Geometry check sheet. Reference: the model listing, model coordinates, mm. A direction names the side the tool comes from. Round coordinates to 2 decimals unless told otherwise and drop trailing zeros. Order: outer loops, then holes, each group sorted by start corner. A loop starts at its lowest first (then second) coordinate and runs counter-clockwise, first axis right, second up. Notation, with made-up numbers: (5.5, 47.5) - (56.5, 47.5) arc R21 ccw to (56.5, 83.5) - close; hole circle Ø2 at (9.25, 89.25). An arc over 180 degrees is marked (long way). Use a Markdown table: item, result. Add a question column.
(1) Section check A-A on z = 10.5. Record the boundary of the cut face in (x, y).
(2) Section check B-B on z = 8. Record the boundary of the cut face in (x, y).
(3) Thickness scan on line 1 along Z through (x, y) = (-7, -20); line 2 along Z through (x, y) = (-6.5, -34.25); line 3 along X through (y, z) = (-23, 2.5). Record the ranges inside material, lowest first. Write a range as [from, to].
(4) Mould release check, pull along Y, two halves, no side actions. Record for faces 3 (the face through (-6.44, -37.03, 6.76)), 4 (the face through (-5.53, -17.68, 4.18)), 5 (the face through (0, -22, 5)): released by +Y, released by -Y, zero draft, split by the parting line, or undercut.
(5) Access from +Z, -Z, +X, -X, +Y, -Y to the whole of each face (thin tool, end or side, straight path). Record for faces 1 (the face through (-5.39, -20.03, 1.01)), 2 (the face through (-8, -21.98, 5.31)).
(6) Gauge pin test, flat ends, axial feed: P1, Ø2, axis at x = -8, z = 4.5, coming from the -Y side; P2, Ø1.5, axis at x = -10, z = 6.5, coming from the -Y side; P3, Ø3, axis at x = -10, y = -34, coming from the +Z side. Record the tip position at first contact, or that the pin passes through.
```python
from build123d import *

# Parameters (mm, degrees)
F0_R     = 5.8053181287
F2_ANGLE = 20
F4_ANGLE = 10
F5_R     = 1.4002438662


with BuildPart() as f2:
    # F0 (on Right) → F2 (revolve)
    with BuildSketch(Plane.YZ):
        with BuildLine():
            Line((-32.5852286816, 0), (-12.5, 0))
            Line((-12.5, 0), (-11.0429839557, 5.8568340727))
            Line((-11.0429839557, 5.8568340727), (-30.835461438, 13.2508232685))
            ThreePointArc((-30.835461438, 13.2508232685), (-35.4357693129, 12.6748361661), (-37.5852286816, 8.5669878109))
            Line((-37.5852286816, 8.5669878109), (-37.5852286816, 5))
            ThreePointArc((-37.5852286816, 5), (-36.1207625875, 1.4644660941), (-32.5852286816, 0))
        make_face()
        with Locations((-31.1660505831, 6.6100014374)):
            Circle(F0_R, mode=Mode.SUBTRACT)
    revolve(axis=Axis((0, 0, 4.1237957776), (0, 0, -1)), revolution_arc=F2_ANGLE)

    # F3 (on face) → F4 (revolve, cut)
    with BuildSketch(Plane(origin=(0, 0, 0), x_dir=(-0.3420201433, -0.9396926208, 0), z_dir=(-0.9396926208, 0.3420201433, 0))):
        with BuildLine():
            Line((12.3108689231, 0.7602588451), (28.9381639648, 1.2491955472))
            ThreePointArc((28.9381639648, 1.2491955472), (26.6792086534, 2.9262576795), (25.4740637742, 5.4685091058))
            Line((25.4740637742, 5.4685091058), (11.7714919778, 2.9284170363))
            Line((11.7714919778, 2.9284170363), (12.3108689231, 0.7602588451))
        make_face()
    revolve(axis=Axis((0, 0, 4.1237957776), (0, 0, 1)), revolution_arc=F4_ANGLE, mode=Mode.SUBTRACT)

    # F5
    f5_edges = [f2.edges().sort_by_distance(p)[0] for p in [
        (-3.233811, -18.339856, 4.198463),
    ]]
    fillet(f5_edges, radius=F5_R)


solid = f2.part
```
Check sheet entries:
| question | item | result |
|---|---|---|
| 1 | outline | (-12.72, -34.95) arc R37.2 ccw to (0, -37.2) - (0, -35.48) arc R35.48 cw to (-12.13, -33.34) - close; (-9.19, -25.24) arc R26.86 ccw to (0, -26.86) - (0, -23.47) arc R23.47 cw to (-8.03, -22.06) - close |
| 2 | outline | (-12.85, -35.32) arc R37.59 ccw to (0, -37.59) - (0, -36.8) arc R36.8 cw to (-12.59, -34.58) - close; (-8.73, -23.99) arc R25.53 ccw to (0, -25.53) - (0, -16.78) arc R16.78 cw to (-5.74, -15.77) - close |
| 3 | line 1 | z = [0, 1.02], [4.67, 9.65] |
| 3 | line 2 | z = [0.55, 2.13], [11.09, 13.02] |
| 3 | line 3 | x = [-4.06, 0] |
| 4 | face 3 | released by -Y |
| 4 | face 4 | undercut |
| 4 | face 5 | zero draft |
| 5 | face 1 | +Y |
| 5 | face 2 | +Z, -Z, -X, +Y |
| 6 | P1 | stops at y = -36.92 |
| 6 | P2 | stops at y = -36.43 |
| 6 | P3 | stops at z = 13.38 |
